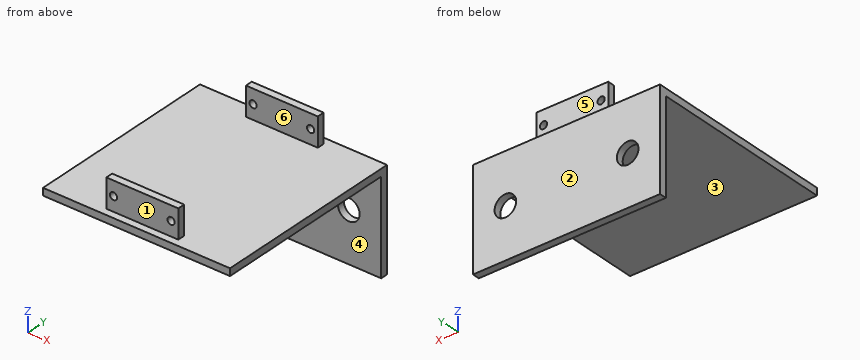
```python
from build123d import *

# Parameters (mm, degrees)
F0_W     = 130
F0_H     = 70
F0_R     = 7.5
F1_DEPTH = 5
F2_W     = 130
F2_H     = 5
F3_DEPTH = 130
F4_W     = 50
F4_H     = 5
F5_DEPTH = 20
F6_R     = 2.5
F7_DEPTH = 130.001


with BuildPart() as f1:
    # F0 (on Front) → F1 (new body)
    with BuildSketch(Plane.XZ):
        with Locations((65, 35)):
            Rectangle(F0_W, F0_H)
        with Locations((22.5, 35)):
            Circle(F0_R, mode=Mode.SUBTRACT)
        with Locations((107.5, 35)):
            Circle(F0_R, mode=Mode.SUBTRACT)
    extrude(amount=F1_DEPTH)

    # F2 (on face) → F3 (join)
    with BuildSketch(Plane.XZ.offset(5)):
        with Locations((65, 67.5)):
            Rectangle(F2_W, F2_H)
    extrude(amount=F3_DEPTH)

    # F4 (on face) → F5 (join)
    with BuildSketch(Plane.XY.offset(70)):
        with Locations((65, -127.5)):
            Rectangle(F4_W, F4_H)
        with Locations((65, -7.5)):
            Rectangle(F4_W, F4_H)
    extrude(amount=F5_DEPTH)

    # F6 (on face) → F7 (cut, through all)
    with BuildSketch(Plane.XZ.offset(130)):
        with Locations((45, 80)):
            Circle(F6_R)
        with Locations((85, 80)):
            Circle(F6_R)
    extrude(amount=-F7_DEPTH, mode=Mode.SUBTRACT)


solid = f1.part
```
Could you check a few things on this model? Use its own coordinates, in mm. Face numbers are marked on the shaded views. A direction names the side the tool comes from. Round coordinates to 2 decimals unless told otherwise and drop trailing zeros. Loops run counter-clockwise (first coordinate to the right, second up) from the corner with the lowest first, then second, coordinate; pieces in that order, holes last. Notation, with made-up numbers: (61.5, 61.5) -> (82.5, 61.5) arc R34 ccw to (82.5, 99.5) -> close; hole circle Ø4 at (1, 52). An arc over 180 degrees is marked (long way). One line per question, with ' | ' between items.
(1) If we section it at D-D on z = 25.5: List the corners of the cut face in (x, y) for me.
Model answer:
outline: (0, -5) -> (130, -5) -> (130, 0) -> (0, 0) -> close
(2) If we section it at A-A on x = 45: List the corners of the cut face in (y, z) for me.
Model answer:
outline: (-135, 65) -> (-5, 65) -> (-5, 0) -> (0, 0) -> (0, 70) -> (-5, 70) -> (-5, 77.5) -> (-10, 77.5) -> (-10, 70) -> (-125, 70) -> (-125, 77.5) -> (-130, 77.5) -> (-130, 70) -> (-135, 70) -> close; (-130, 82.5) -> (-125, 82.5) -> (-125, 90) -> (-130, 90) -> close; (-10, 82.5) -> (-5, 82.5) -> (-5, 90) -> (-10, 90) -> close
(3) For pin 1 Ø1 at (x, y) = (113.5, -73) entering from +Z; pin 2 Ø6 at (x, z) = (71.5, 76.5) entering from +Y; pin 3 Ø19.5 at (x, z) = (84.5, 28.5) entering from -Y, each with a flat end and sliding along its axis, tell me the tip position at first contact or that it passes through.
Model answer:
pin 1: stops at z = 70 | pin 2: stops at y = -5 | pin 3: stops at y = -5
(4) If we section it at C-C on x = 22.5: List the corners of the cut face in (y, z) for me.
Model answer:
outline: (-135, 65) -> (-5, 65) -> (-5, 42.5) -> (0, 42.5) -> (0, 70) -> (-135, 70) -> close; (-5, 0) -> (0, 0) -> (0, 27.5) -> (-5, 27.5) -> close
(5) If I drill on probe 1 along Z at (x, y) = (22.5, -3.55); probe 2 along Z at (x, y) = (45, -128.6); probe 3 along Y at (x, z) = (80, 84.5), over which ranges is the centre line in solid material (lowest first)?
Model answer:
probe 1: z = 0 to 27.5, 42.5 to 70 | probe 2: z = 65 to 77.5, 82.5 to 90 | probe 3: y = -130 to -125, -10 to -5
(6) If we section it at B-B on z = 35: List the corners of the cut face in (x, y) for me.
Model answer:
outline: (0, -5) -> (15, -5) -> (15, 0) -> (0, 0) -> close; (30, -5) -> (100, -5) -> (100, 0) -> (30, 0) -> close; (115, -5) -> (130, -5) -> (130, 0) -> (115, 0) -> close
(7) For the marked faces 1, 2 and 3, which set-ups out of +Z, -Z, +X, -X, +Y, -Y let a thin tool reach every point of the face, with its end or its side?
Model answer:
face 1: +Z, +X, -X, -Y | face 2: +Z, -Z, +X, -X, +Y | face 3: -Z, +X, -X, -Y
(8) Thinking about a two-plate mould opening in Y: for the marked faces 4, 5 and 6, which applies, released by +Y, released by -Y, zero draft, split by the parting line, or undercut?
Model answer:
face 4: released by -Y | face 5: released by +Y | face 6: undercut
